from build123d import *

# Parameters (mm, degrees)
SKETCH_1_W          = 20
SKETCH_1_H          = 20
EXTRUDE_1_DEPTH     = 3
SKETCH_2_W          = 2
SKETCH_2_H          = 20
EXTRUDE_2_DEPTH     = 20
CUT_EXTRUDE_START   = -14
CUT_EXTRUDE_2_DEPTH = 14
SKETCH_4_R          = 2
CUT_EXTRUDE_3_DEPTH = 31.298514815
SKETCH_6_R          = 4
CUT_EXTRUDE_5_DEPTH = 25.494897428
SKETCH_7_W          = 8.2
SKETCH_7_H          = 1
EXTRUDE_3_DEPTH     = 2


# Read off the part's stored shape, not the designer's step: 切除-拉伸2
with BuildPart() as part:
    # 草图1 → 凸台-拉伸1 (new body)
    with BuildSketch(Plane.XY):
        Rectangle(SKETCH_1_W, SKETCH_1_H)
    extrude(amount=EXTRUDE_1_DEPTH)

    # 草图2 → 凸台-拉伸2 (add)
    with BuildSketch(Plane.XY.offset(3)):
        with Locations((-6, 0)):
            Rectangle(SKETCH_2_W, SKETCH_2_H)
        with Locations((6, 0)):
            Rectangle(SKETCH_2_W, SKETCH_2_H)
    extrude(amount=EXTRUDE_2_DEPTH)

    # 切除-拉伸2 outline → 切除-拉伸2 (cut)
    with BuildSketch(Plane.ZY.offset(7).offset(CUT_EXTRUDE_START)):
        with BuildLine():
            Line((23, 10), (13, 10))
            ThreePointArc((13, 10), (20.071067812, 7.071067812), (23, 0))
            Line((23, 0), (23, 10))
        make_face()
        with BuildLine():
            Line((23, -10), (23, 0))
            ThreePointArc((23, 0), (20.071067812, -7.071067812), (13, -10))
            Line((13, -10), (23, -10))
        make_face()
    extrude(amount=CUT_EXTRUDE_2_DEPTH, mode=Mode.SUBTRACT)

    # 草图4 → 切除-拉伸3 (cut, through all)
    with BuildSketch(Plane.ZY.offset(7)):
        with Locations((13, 0)):
            Circle(SKETCH_4_R)
    extrude(amount=-CUT_EXTRUDE_3_DEPTH, mode=Mode.SUBTRACT)

    # 草图6 → 切除-拉伸5 (cut, through all)
    with BuildSketch(Plane.XY.offset(3)):
        Circle(SKETCH_6_R)
    extrude(amount=-CUT_EXTRUDE_5_DEPTH, mode=Mode.SUBTRACT)

    # 草图7 → 凸台-拉伸3 (add)
    with BuildSketch(Plane(origin=(0, 0, 0), x_dir=(-1, 0, 0), z_dir=(0, 0, -1))):
        with Locations((0, 9.5)):
            Rectangle(SKETCH_7_W, SKETCH_7_H)
        with Locations((0, -9.5)):
            Rectangle(SKETCH_7_W, SKETCH_7_H)
    extrude(amount=EXTRUDE_3_DEPTH)


solid = part.part
The listing builds one solid part. Answer for the finished solid, in the listing's coordinates (mm). A direction names the side the tool comes from. Coordinates: 2 decimals unless noted, no trailing zeros. Loops run counter-clockwise (first coordinate to the right, second up) from the corner with the lowest first, then second, coordinate; pieces in that order, holes last.
1) A tool of negligible diameter and unlimited length cuts with its end or side. For faces 5 (the face through (5, -0.1, 10.6)), 6 (the face through (4.1, -9.5, -1)), 7 (the face through (-7, -0.1, 10.6)), 8 (the face through (8, 0, 3)), from which of +Z, -Z, +X, -X, +Y, -Y can it reach the whole face along a straight path? Write none if from no direction.
2) Determine the mould class of faces 1 (the face through (-6, -1.2, 11.4)), 2 (the face through (0.1, 9.5, -2)), 3 (the face through (-9, 0, 3)), 4 (the face through (-4.1, -9.5, -1)) for opening direction Z: pulls with the +Z half, pulls with the -Z half, needs draft (parallel to the pull), parting line crosses it, or undercut.
3) Find section A-A on y = -2.5. Write down the section's boundary in (x, z), then the cut area to 3 significant figures.
4) Find section D-D on z = 13.75. Write down the section's boundary in (x, y), then the cut area to 3 significant figures.
5) Find section B-B on z = 16.75. Write down the section's boundary in (x, y).
6) Flat-ended cylindrical pins translate along their axes: pin 1 Ø2 at (y, z) = (2, 5) entering from +X; pin 2 Ø0.9 at (x, y) = (-8, -4) entering from +Z; pin 3 Ø5 at (x, z) = (4, 8) entering from -Y; pin 4 Ø6 at (x, y) = (-3, 0) entering from -Z. Find the tip coordinate at first contact, or state that the pin passes through.
7) Find section C-C on x = 3.25. Write down the section's boundary in (y, z), then the cut area to 3 significant figures.
8) Find the intervals of material crossed by L1, parallel to X at y = 6.25, z = 9.75; L2, parallel to Y at x = -5.4, z = 13; L3, parallel to Y at x = 0, z = 1.5, in increasing order.
Values:
1. face 5: +Z, +Y, -Y
1. face 6: -Z, +X, +Y, -Y
1. face 7: +Z, -X, +Y, -Y
1. face 8: +Z, +X, +Y, -Y
2. face 1: undercut
2. face 2: pulls with the -Z half
2. face 3: pulls with the +Z half
2. face 4: needs draft
3. outline: (-10, 0) - (-3.12, 0) - (-3.12, 3) - (-5, 3) - (-5, 22.68) - (-7, 22.68) - (-7, 3) - (-10, 3) - close; (3.12, 0) - (10, 0) - (10, 3) - (7, 3) - (7, 22.68) - (5, 22.68) - (5, 3) - (3.12, 3) - close
3. area: 120 mm2
4. outline: (-7, -9.97) - (-5, -9.97) - (-5, -1.85) - (-7, -1.85) - close; (-7, 1.85) - (-5, 1.85) - (-5, 9.97) - (-7, 9.97) - close; (5, -9.97) - (7, -9.97) - (7, -1.85) - (5, -1.85) - close; (5, 1.85) - (7, 1.85) - (7, 9.97) - (5, 9.97) - close
4. area: 64.9 mm2
5. outline: (-7, -9.27) - (-5, -9.27) - (-5, 9.27) - (-7, 9.27) - close; (5, -9.27) - (7, -9.27) - (7, 9.27) - (5, 9.27) - close
6. pin 1: stops at x = 7
6. pin 2: stops at z = 3
6. pin 3: stops at y = -10
6. pin 4: stops at z = 0
7. outline: (-10, -2) - (-9, -2) - (-9, 0) - (-2.33, 0) - (-2.33, 3) - (-10, 3) - close; (2.33, 0) - (9, 0) - (9, -2) - (10, -2) - (10, 3) - (2.33, 3) - close
7. area: 50.0 mm2
8. L1: x = -7 to -5, 5 to 7
8. L2: y = -10 to -2, 2 to 10
8. L3: y = -10 to -4, 4 to 10
